Verification items for the finished model (mm, model axes). Coordinates: 2 decimals unless noted, no trailing zeros. Order: outer loops, then holes, each group sorted by start corner. A loop starts at its lowest first (then second) coordinate and runs counter-clockwise, first axis right, second up. Notation, with made-up numbers: M -20,-5.5 L -11,-5.5 A32 cw -11,22.5 Z; hole C 68.25,75 d10. An arc over 180 degrees is marked long. Return JSON: item names as keys, results as strings. Group by question number.
Q1. Section check B-B, the plane x = -122. Enter the section's corners in (y, z), then the cut area to 3 significant figures.
Q2. Section check A-A, the plane y = 1877.5. Enter the section's corners in (x, z).
Q3. Thickness scan on probe 1 along Y at (x, z) = (228.6, 4.25); probe 2 along Y at (x, z) = (90, 4); probe 3 along X at (y, z) = (1600.2, 2.5). Record the ranges inside material, lowest first.
Q4. Section check C-C, the plane z = 3.25. Count the separate pieces of the cut face and the enclosed holes in it, then the cut area to 3 significant figures.
Q5. Mould release check, pull along X, two halves, no side actions. Record for faces 1 (the face through (209.527, 1899.337, 3.131)), 2 (the face through (-182, 2050, 0)), 3 (the face through (-209.527, 1905.583, 3.131)): pulls with the +X half, pulls with the -X half, needs draft (parallel to the pull), parting line crosses it, or undercut.
Q6. Go/stop test with flat-tipped pins: pin 1 Ø9 at (x, y) = (-190.5, 2104.78) entering from +Z; pin 2 Ø1 at (x, z) = (14.5, 3.5) entering from -Y; pin 3 Ø7 at (x, y) = (-190.5, 2200.03) entering from -Z (1 decimal); pin 4 Ø3 at (y, z) = (1524, 2.5) entering from +X. Record where each tip stops, or that it passes through.
from build123d import *

# Parameters (mm, degrees)
SKETCH1_W                      = 533.4
SKETCH1_H                      = 2413
BOSS_EXTRUDE1_DEPTH            = 6.35
F_5_16_0_3125_DIAMETER_HOLE1_D = 7.9375
SKETCH6_W                      = 533.4
SKETCH6_H                      = 1546.86
CUT_EXTRUDE1_DEPTH             = 7.35
SKETCH7_W                      = 62.992
SKETCH7_H                      = 38.1
BOSS_EXTRUDE2_DEPTH            = 6.35
FILLET1_R                      = 6.35
SKETCH9_W                      = 533.4
SKETCH9_H                      = 27.94
CUT_EXTRUDE3_DEPTH             = 7.35
F_5_16_0_3125_DIAMETER_HOLE2_D = 7.9375


with BuildPart() as part:
    # Sketch1 → Boss-Extrude1 (new body)
    with BuildSketch(Plane.XY):
        with Locations((0, 1206.5)):
            Rectangle(SKETCH1_W, SKETCH1_H)
        with BuildLine():
            Line((-101.6, 797.56), (101.6, 797.56))
            Line((101.6, 797.56), (101.6, 663.332045059))
            ThreePointArc((101.6, 663.332045059), (209.55, 480.06), (101.6, 296.787954941))
            Line((101.6, 296.787954941), (101.6, 162.56))
            Line((101.6, 162.56), (-101.6, 162.56))
            Line((-101.6, 162.56), (-101.6, 296.787954941))
            ThreePointArc((-101.6, 296.787954941), (-209.55, 480.06), (-101.6, 663.332045059))
            Line((-101.6, 663.332045059), (-101.6, 797.56))
        make_face(mode=Mode.SUBTRACT)
        with BuildLine():
            Line((-101.6, 1508.76), (-101.6, 1374.532045059))
            ThreePointArc((-101.6, 1374.532045059), (-209.55, 1191.26), (-101.6, 1007.987954941))
            Line((-101.6, 1007.987954941), (-101.6, 873.76))
            Line((-101.6, 873.76), (101.6, 873.76))
            Line((101.6, 873.76), (101.6, 1007.987954941))
            ThreePointArc((101.6, 1007.987954941), (209.55, 1191.26), (101.6, 1374.532045059))
            Line((101.6, 1374.532045059), (101.6, 1508.76))
            Line((101.6, 1508.76), (-101.6, 1508.76))
        make_face(mode=Mode.SUBTRACT)
        with BuildLine():
            Line((-101.6, 2219.96), (-101.6, 2085.732045059))
            ThreePointArc((-101.6, 2085.732045059), (-209.55, 1902.46), (-101.6, 1719.187954941))
            Line((-101.6, 1719.187954941), (-101.6, 1584.96))
            Line((-101.6, 1584.96), (101.6, 1584.96))
            Line((101.6, 1584.96), (101.6, 1719.187954941))
            ThreePointArc((101.6, 1719.187954941), (209.55, 1902.46), (101.6, 2085.732045059))
            Line((101.6, 2085.732045059), (101.6, 2219.96))
            Line((101.6, 2219.96), (-101.6, 2219.96))
        make_face(mode=Mode.SUBTRACT)
    extrude(amount=BOSS_EXTRUDE1_DEPTH)

    # 5/16 (0.3125) Diameter Hole1 (through all)
    with Locations(Plane.XY.offset(6.35)):
        with Locations((-76.2, 146.685), (-76.2, 102.235), (-228.6, 177.8), (76.2, 102.235), (76.2, 146.685), (-76.2, 857.885), (-76.2, 813.435), (76.2, 813.435), (76.2, 857.885), (-76.2, 1569.085), (-76.2, 1524.635), (76.2, 1524.635), (76.2, 1569.085), (228.6, 177.8), (-228.6, 889), (228.6, 889), (-228.6, 1600.2), (228.6, 1600.2), (0, 2280.285), (0, 2235.835), (228.6, 2311.4), (-228.6, 2311.4)):
            Hole(F_5_16_0_3125_DIAMETER_HOLE1_D / 2)

    # Sketch6 → Cut-Extrude1 (cut, through all)
    with BuildSketch(Plane.XY.offset(6.35)):
        with Locations((0, 773.43)):
            Rectangle(SKETCH6_W, SKETCH6_H)
    extrude(amount=-CUT_EXTRUDE1_DEPTH, mode=Mode.SUBTRACT)

    # Sketch7 → Boss-Extrude2 (add)
    with BuildSketch(Plane.XY.offset(6.35)):
        with Locations((-184.15, 1527.81)):
            Rectangle(SKETCH7_W, SKETCH7_H)
        with Locations((184.15, 1527.81)):
            Rectangle(SKETCH7_W, SKETCH7_H)
    extrude(amount=-BOSS_EXTRUDE2_DEPTH)

    # Fillet1
    fillet1_edges = [part.edges().sort_by_distance(p)[0] for p in [
        (-152.654, 1508.76, 3.175),
        (-215.646, 1508.76, 3.175),
        (-215.646, 1546.86, 3.175),
        (-152.654, 1546.86, 3.175),
        (215.646, 1508.76, 3.175),
        (215.646, 1546.86, 3.175),
        (152.654, 1546.86, 3.175),
        (152.654, 1508.76, 3.175),
    ]]
    fillet(fillet1_edges, radius=FILLET1_R)

    # Sketch9 → Cut-Extrude3 (cut, through all)
    with BuildSketch(Plane.XY.offset(6.35)):
        with Locations((0, 2399.03)):
            Rectangle(SKETCH9_W, SKETCH9_H)
    extrude(amount=-CUT_EXTRUDE3_DEPTH, mode=Mode.SUBTRACT)

    # 5/16 (0.3125) Diameter Hole2 (through all)
    with Locations(Plane.XY.offset(6.35)):
        with Locations((-190.5, 2200.032045059), (-190.5, 2104.782045059), (190.5, 2200.032045059), (190.5, 2104.782045059)):
            Hole(F_5_16_0_3125_DIAMETER_HOLE2_D / 2)


solid = part.part
Numbers:
{
 "1": {"outline": "M 1546.86,0 L 1732.09,0 L 1732.09,6.35 L 1546.86,6.35 Z; M 2072.83,0 L 2385.06,0 L 2385.06,6.35 L 2072.83,6.35 Z", "area": "3,160 mm2"},
 "2": {"outline": "M -266.7,0 L -208.06,0 L -208.06,6.35 L -266.7,6.35 Z; M 208.06,0 L 266.7,0 L 266.7,6.35 L 208.06,6.35 Z"},
 "3": {"probe 1": "y = 1546.86 to 1596.23, 1604.17 to 2307.43, 2315.37 to 2385.06", "probe 2": "y = 1546.86 to 1584.96, 2219.96 to 2385.06", "probe 3": "x = -266.7 to -232.57, -224.63 to -101.6, 101.6 to 224.63, 232.57 to 266.7"},
 "4": {"separate pieces": "1", "enclosed holes": "13", "area": "266,000 mm2"},
 "5": {"face 1": "undercut", "face 2": "needs draft", "face 3": "undercut"},
 "6": {"pin 1": "stops at z = 6.35", "pin 2": "stops at y = 1546.86", "pin 3": "passes through", "pin 4": "stops at x = 215.65"}
}
